from build123d import *

# Parameters (mm, degrees)
BOSS_EXTRUDE1_DEPTH     = 10
CUT_EXTRUDE1_DEPTH      = 72.414284285
CUT_EXTRUDE1_DEPTH_BACK = 72.414284285
SKETCH2_R               = 1.5
SKETCH9_W               = 10
SKETCH9_H               = 50
BOSS_EXTRUDE9_DEPTH     = 5
SKETCH10_W              = 10
SKETCH10_H              = 50
BOSS_EXTRUDE10_DEPTH    = 5
BOSS_EXTRUDE11_DEPTH    = 2
SKETCH12_W              = 10
SKETCH12_H              = 10
BOSS_EXTRUDE12_DEPTH    = 5
CUT_EXTRUDE2_START      = 7
SKETCH13_R              = 1.5
CUT_EXTRUDE2_DEPTH      = 7
BOSS_EXTRUDE13_DEPTH    = 2
SKETCH15_W              = 9.981523119
SKETCH15_H              = 10
BOSS_EXTRUDE14_DEPTH    = 30
SKETCH16_R              = 1.5
CUT_EXTRUDE3_DEPTH      = 32
SKETCH18_W              = 10
SKETCH18_H              = 89
BOSS_EXTRUDE15_DEPTH    = 30
SKETCH19_W              = 5
SKETCH19_H              = 89
BOSS_EXTRUDE16_DEPTH    = 15
FILLET1_R               = 5
SKETCH20_R              = 2.48436703
SKETCH20_R_2            = 2
CUT_EXTRUDE4_DEPTH      = 149.657324071
SKETCH22_R              = 2
CUT_EXTRUDE5_DEPTH      = 104.435970532


with BuildPart() as part:
    # Sketch1 → Boss-Extrude1 (new body)
    with BuildSketch(Plane.XY):
        with BuildLine():
            Line((45.018476881, -25), (50, -25))
            Line((50, -25), (50, 25))
            Line((50, 25), (45, 25))
            ThreePointArc((45, 25), (0, 8), (-45, 25))
            Line((-45, 25), (-50, 25))
            Line((-50, 25), (-50, -25))
            Line((-50, -25), (-45.018476881, -25))
            ThreePointArc((-45.018476881, -25), (0, -8), (45.018476881, -25))
        make_face()
    extrude(amount=BOSS_EXTRUDE1_DEPTH)

    # Sketch2 → Cut-Extrude1 (cut, two sides: drawn at the far end of the back side and taken through both)
    with BuildSketch(Plane(origin=(0, 25, 0), x_dir=(1, 0, 0), z_dir=(0, 1, 0)).offset(-CUT_EXTRUDE1_DEPTH_BACK)):
        with Locations(Location((-48, -5, 0), (0, 0, 180))):
            Circle(SKETCH2_R)
        with Locations(Location((48, -5, 0), (0, 0, 180))):
            Circle(SKETCH2_R)
    extrude(amount=CUT_EXTRUDE1_DEPTH + CUT_EXTRUDE1_DEPTH_BACK, mode=Mode.SUBTRACT)

    # Sketch9 → Boss-Extrude9 (add)
    with BuildSketch(Plane(origin=(50, 0, 0), x_dir=(0, 0, -1), z_dir=(1, 0, 0))):
        with Locations((-5, 0)):
            Rectangle(SKETCH9_W, SKETCH9_H)
    extrude(amount=BOSS_EXTRUDE9_DEPTH)

    # Sketch10 → Boss-Extrude10 (add)
    with BuildSketch(Plane.ZY.offset(50)):
        with Locations((5, 0)):
            Rectangle(SKETCH10_W, SKETCH10_H)
    extrude(amount=BOSS_EXTRUDE10_DEPTH)

    # Sketch11 → Boss-Extrude11 (add)
    with BuildSketch(Plane(origin=(0, 25, 0), x_dir=(1, 0, 0), z_dir=(0, 1, 0))):
        Polygon((50, 0), (50, -7), (45, -7), (45, -10), (55, -10), (55, 0), align=None)
        Polygon((-50, 0), (-50, -7), (-45, -7), (-45, -10), (-55, -10), (-55, 0), align=None)
    extrude(amount=BOSS_EXTRUDE11_DEPTH)

    # Sketch12 → Boss-Extrude12 (add)
    with BuildSketch(Plane(origin=(0, 27, 0), x_dir=(1, 0, 0), z_dir=(0, 1, 0))):
        with Locations((50, -5)):
            Rectangle(SKETCH12_W, SKETCH12_H)
        with Locations((-50, -5)):
            Rectangle(SKETCH12_W, SKETCH12_H)
    extrude(amount=BOSS_EXTRUDE12_DEPTH)

    # Sketch13 → Cut-Extrude2 (cut)
    with BuildSketch(Plane(origin=(0, 25, 0), x_dir=(1, 0, 0), z_dir=(0, 1, 0)).offset(CUT_EXTRUDE2_START)):
        with Locations(Location((48, -5, 0), (0, 0, 180))):
            Circle(SKETCH13_R)
        with Locations(Location((-48, -5, 0), (0, 0, 180))):
            Circle(SKETCH13_R)
    extrude(amount=-CUT_EXTRUDE2_DEPTH, mode=Mode.SUBTRACT)

    # Sketch14 → Boss-Extrude13 (add)
    with BuildSketch(Plane.XZ.offset(25)):
        Polygon((50.009238441, 0), (50.009238441, 7), (45.018476881, 7), (45.018476881, 10), (55, 10), (55, 0), align=None)
        Polygon((-50.009238441, 0), (-50.009238441, 7), (-45.018476881, 7), (-45.018476881, 10), (-55, 10), (-55, 0), align=None)
    extrude(amount=BOSS_EXTRUDE13_DEPTH)

    # Sketch15 → Boss-Extrude14 (add)
    with BuildSketch(Plane.XZ.offset(27)):
        with Locations((-50.00923844, 5)):
            Rectangle(SKETCH15_W, SKETCH15_H)
        with Locations((50.00923844, 5)):
            Rectangle(SKETCH15_W, SKETCH15_H)
    extrude(amount=BOSS_EXTRUDE14_DEPTH)

    # Sketch16 → Cut-Extrude3 (cut)
    with BuildSketch(Plane.XZ.offset(25)):
        with Locations(Location((48, 5, 0), (0, 0, 180))):
            Circle(SKETCH16_R)
        with Locations(Location((-48, 5, 0), (0, 0, 180))):
            Circle(SKETCH16_R)
    extrude(amount=CUT_EXTRUDE3_DEPTH, mode=Mode.SUBTRACT)

    # Sketch18 → Boss-Extrude15 (add)
    with BuildSketch(Plane(origin=(55, 0, 0), x_dir=(0, 0, -1), z_dir=(1, 0, 0))):
        with Locations((-5, -12.5)):
            Rectangle(SKETCH18_W, SKETCH18_H)
    extrude(amount=BOSS_EXTRUDE15_DEPTH)

    # Sketch19 → Boss-Extrude16 (add)
    with BuildSketch(Plane.XY.offset(10)):
        with Locations((82.5, -12.5)):
            Rectangle(SKETCH19_W, SKETCH19_H)
    extrude(amount=BOSS_EXTRUDE16_DEPTH)

    # Fillet1
    fillet1_edges = [part.edges().sort_by_distance(p)[0] for p in [
        (80, -12.5, 10),
    ]]
    fillet(fillet1_edges, radius=FILLET1_R)

    # Sketch20 → Cut-Extrude4 (cut, through all)
    with BuildSketch(Plane.ZY.offset(-80)):
        with Locations(Location((20, 9.75, 0), (0, 0, 270))):
            Circle(SKETCH20_R)
        with Locations(Location((20, -12.5, 0), (0, 0, 270))):
            Circle(SKETCH20_R_2)
        with Locations(Location((20, -34.75, 0), (0, 0, 270))):
            Circle(SKETCH20_R_2)
    extrude(amount=-CUT_EXTRUDE4_DEPTH, mode=Mode.SUBTRACT)

    # Sketch22 → Cut-Extrude5 (cut, through all)
    with BuildSketch(Plane.XY.offset(10)):
        with Locations((65, 20.875)):
            Circle(SKETCH22_R)
        with Locations((65, -1.375)):
            Circle(SKETCH22_R)
        with Locations((65, -23.625)):
            Circle(SKETCH22_R)
        with Locations((65, -45.875)):
            Circle(SKETCH22_R)
    extrude(amount=-CUT_EXTRUDE5_DEPTH, mode=Mode.SUBTRACT)


solid = part.part
Source: CAD feature listing. Evaluate the final solid. Frame: model axes, mm. A direction names the side the tool comes from. Give positions to 0.01 mm unless a question says otherwise; leave off trailing zeros. Write each loop counter-clockwise with the first axis right and the second up, starting at its lowest first coordinate (ties: lowest second). Pieces come first, ordered by that corner, then holes. Notation, with made-up numbers: (2.25, 66) - (35.25, 66) arc R27 cw to (35.25, 91) - close; hole circle Ø5 at (82, -27.5). An arc over 180 degrees is marked (long way). Write item = value, one per line. Start each with the question number.
Q1. Cut plane B-B, the plane x = 65. Return loops of the section in (y, z) (3 decimals), then the cut area to 3 significant figures.
Q2. Reachability of faces 1 (the flat face through (-48, -27, 3)), 2 (the flat face through (-45.018, -41, 5)), 3 (the cylindrical face through (64.57, -47.83, 5.07)), 4 (the cylindrical face through (82.465, 10.073, 22.463)), 5 (the flat face through (45, 29, 5)) from +Z, -Z, +X, -X, +Y, -Y: full face, straight path, thin tool, end or side. Return the list, or none.
Q3. Cut plane A-A, the plane y = -34.75. Return loops of the section in (x, z), then the cut area to 3 significant figures.
Q4. Draft query along X for faces 6 (the flat face through (-50, 32, 5)), 7 (the cylindrical face through (49.5, -41.79, 4.93)), 8 (the cylindrical face through (79, -12, 12)), 9 (the cylindrical face through (-46.5, -41.79, 4.93)). Return one class per face: +X half, -X half, draft (parallel to the pull), parting line (faces both ways), or undercut.
Q5. Cut plane C-C, the plane x = 48. Return loops of the section in (y, z), then the cut area to 3 significant figures.
Q6. Material intervals for probe 1 along Y at (x, z) = (65, 3.25) (3 decimals); probe 2 along X at (y, z) = (-48.5, 5); probe 3 along Y at (x, z) = (47, 1.25), sorted ascending.
Q7. Pin query (flat end, axial travel): pin 1 Ø8 at (y, z) = (-12, 19) entering from -X; pin 2 Ø1 at (x, z) = (3, 10) entering from -Y; pin 3 Ø8 at (x, y) = (43, -39.5) entering from +Z; pin 4 Ø2.5 at (x, z) = (48, 5) entering from +Y. Return the tip coordinate at first contact, or that it passes through.
Q8. Cut plane D-D, the plane y = 16.5. Return loops of the section in (x, z).
Computed values:
q1.outline = (-57, 0) - (-47.875, 0) - (-47.875, 10) - (-57, 10) - close; (-43.875, 0) - (-25.625, 0) - (-25.625, 10) - (-43.875, 10) - close; (-21.625, 0) - (-3.375, 0) - (-3.375, 10) - (-21.625, 10) - close; (0.625, 0) - (18.875, 0) - (18.875, 10) - (0.625, 10) - close; (22.875, 0) - (32, 0) - (32, 10) - (22.875, 10) - close
q1.area = 730 mm²
q2.face_1 = -Z
q2.face_2 = +Z, -Z, -Y
q2.face_3 = +Z, -Z
q2.face_4 = +X, -X
q2.face_5 = +Z, -Z, +Y
q3.outline = (-55, 0) - (-45.02, 0) - (-45.02, 10) - (-55, 10) - close; (45.02, 0) - (85, 0) - (85, 18) - (80, 18) - (80, 15) arc R5 cw to (75, 10) - (45.02, 10) - close; (80, 22) - (85, 22) - (85, 25) - (80, 25) - close; hole circle Ø3 at (-48, 5); hole circle Ø3 at (48, 5)
q3.area = 546 mm²
q4.face_6 = draft
q4.face_7 = undercut
q4.face_8 = -X half
q4.face_9 = undercut
q5.outline = (-57, 0) - (-27, 0) - (-27, 3.5) - (-57, 3.5) - close; (-57, 6.5) - (-27, 6.5) - (-27, 7) - (-25, 7) - (-25, 6.5) - (25, 6.5) - (25, 7) - (27, 7) - (27, 6.5) - (32, 6.5) - (32, 10) - (-57, 10) - close; (-25, 0) - (25, 0) - (25, 3.5) - (-25, 3.5) - close; (27, 0) - (32, 0) - (32, 3.5) - (27, 3.5) - close
q5.area = 607 mm²
q6.probe_1 = -57 to -47.875, -43.875 to -25.625, -21.625 to -3.375, 0.625 to 18.875, 22.875 to 32
q6.probe_2 = -55 to -49.5, -46.5 to -45.02, 45.02 to 46.5, 49.5 to 85
q6.probe_3 = -57 to -27, -25 to 25, 27 to 32
q7.pin_1 = 80
q7.pin_2 = -8.09
q7.pin_3 = 10
q7.pin_4 = through
q8.outline = (-55, 0) - (-32.94, 0) - (-32.94, 10) - (-55, 10) - close; (32.94, 0) - (85, 0) - (85, 25) - (80, 25) - (80, 15) arc R5 cw to (75, 10) - (32.94, 10) - close; hole circle Ø3 at (-48, 5); hole circle Ø3 at (48, 5)
